Check sheet for the modelled part. Datum: model origin and axes. Units: mm. Face numbers are marked on the shaded views. A direction names the side the tool comes from. Round coordinates to 2 decimals unless told otherwise and drop trailing zeros. Write each loop counter-clockwise with the first axis right and the second up, starting at its lowest first coordinate (ties: lowest second). Pieces come first, ordered by that corner, then holes.
Item 1: Section check B-B, the plane z = -27. Record the cut outline in (x, y), plus the area to 3 significant figures.
Item 2: Section check C-C, the plane x = 15. Record the cut outline in (y, z).
Item 3: Depth check by flat-ended pin: pin 1 (1.2 mm diameter, centred on x = 7, y = 0.5, fed in from -Z); pin 2 (4 mm diameter, centred on x = -18, z = 5, fed in from +Y); pin 3 (1 mm diameter, centred on y = 9.5, z = -1.5, fed in from -X). Enter the tip coordinate at first touch or a pass-through.
Item 4: Material ranges on line 1 along Y through (x, z) = (0, 16); line 2 along Y through (x, z) = (-47, -10.5); line 3 along Z through (x, y) = (-6, 21.25), recorded low to high.
Item 5: Release check for a two-part mould opening along X. For the marked faces 3, 4, 5 and 6 record: pulls with the +X half, pulls with the -X half, needs draft (parallel to the pull), parting line crosses it, or undercut.
Item 6: Section check D-D, the plane y = 25.75. Record the cut outline in (x, z), plus the area to 3 significant figures.
Item 7: Section check A-A, the plane x = 0. Record the cut outline in (y, z).
Item 8: Set-up check for the marked faces 1 and 2: record each of +Z, -Z, +X, -X, +Y, -Y from which the full face is reachable in a straight line by a thin tool's end or side.
from build123d import *

# Parameters (mm, degrees)
SALIENTE_EXTRUIR1_DEPTH = 1.5
SALIENTE_EXTRUIR2_DEPTH = 30
CROQUIS3_R              = 8.9
CORTAR_EXTRUIR1_DEPTH   = 30
CROQUIS4_R              = 8.9
CORTAR_EXTRUIR2_DEPTH   = 30
CROQUIS5_R              = 8.9
CORTAR_EXTRUIR3_DEPTH   = 30


with BuildPart() as part:
    # Croquis1 → Saliente-Extruir1 (new body)
    with BuildSketch(Plane(origin=(0, 0, 0), x_dir=(1, 0, 0), z_dir=(0, 1, 0))):
        Polygon((-19, -15), (-51.571428571, 4.572992638), (-36.119065962, 30.287278353), (-19, 20), (-19, 15), (19, 15), (19, 20), (36.119065962, 30.287278353), (51.571428571, 4.572992638), (19, -15), align=None)
    extrude(amount=SALIENTE_EXTRUIR1_DEPTH)

    # Croquis2 → Saliente-Extruir2 (add)
    with BuildSketch(Plane(origin=(0, 0, 0), x_dir=(1, 0, 0), z_dir=(0, 1, 0))):
        Polygon((-51.571428571, 4.572992638), (-52.344046702, 3.287278353), (-19.416025147, -16.5), (19.416025147, -16.5), (52.344046702, 3.287278353), (51.571428571, 4.572992638), (19, -15), (-19, -15), align=None)
    extrude(amount=SALIENTE_EXTRUIR2_DEPTH)

    # Croquis3 → Cortar-Extruir1 (cut)
    with BuildSketch(Plane.XY.offset(16.5)):
        with Locations((0, 14.563888597)):
            Circle(CROQUIS3_R)
    extrude(amount=-CORTAR_EXTRUIR1_DEPTH, mode=Mode.SUBTRACT)

    # Croquis4 → Cortar-Extruir2 (cut)
    with BuildSketch(Plane(origin=(12.435875575, 0, 20.694547865), x_dir=(0.8571428571428564, 0, -0.5150787536377139), z_dir=(0.5150787536377139, 0, 0.8571428571428564))):
        with Locations((27.351520408, 15)):
            Circle(CROQUIS4_R)
    extrude(amount=-CORTAR_EXTRUIR2_DEPTH, mode=Mode.SUBTRACT)

    # Croquis5 → Cortar-Extruir3 (cut)
    with BuildSketch(Plane(origin=(-12.435875575, 0, 20.694547865), x_dir=(0.8571428571428567, 0, 0.5150787536377137), z_dir=(-0.5150787536377136, 0, 0.8571428571428565))):
        with Locations((-27.351520408, 15)):
            Circle(CROQUIS5_R)
    extrude(amount=-CORTAR_EXTRUIR3_DEPTH, mode=Mode.SUBTRACT)


solid = part.part
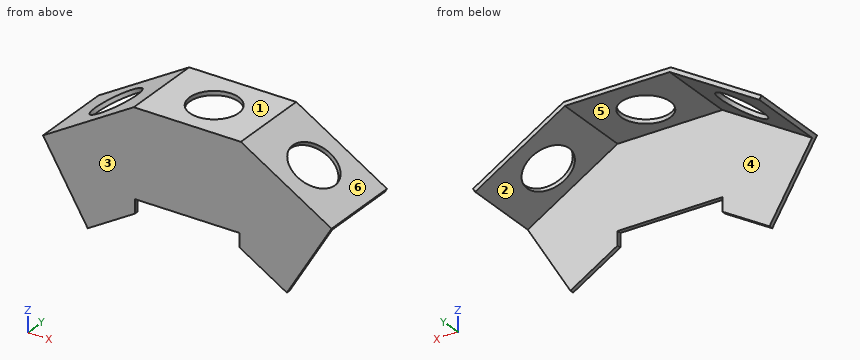
Values found:
1. outline: (-38.09, 0) - (-30.65, 0) - (-30.65, 1.5) - (-38.09, 1.5) - close; (30.65, 0) - (38.09, 0) - (38.09, 1.5) - (30.65, 1.5) - close
1. area: 22.3 mm2
2. outline: (0, -15) - (1.5, -15) - (1.5, 15) - (30, 15) - (30, 16.5) - (0, 16.5) - close
3. pin 1: stops at z = -15
3. pin 2: stops at y = 1.5
3. pin 3: stops at x = -50.2
4. line 1: y = 0 to 5.66, 23.46 to 30
4. line 2: y = 0 to 1.5
4. line 3: z = 15 to 16.5
5. face 3: needs draft
5. face 4: undercut
5. face 5: undercut
5. face 6: pulls with the +X half
6. outline: (-52.34, -3.29) - (-51.57, -4.57) - (-19, 15) - (19, 15) - (51.57, -4.57) - (52.34, -3.29) - (19.42, 16.5) - (-19.42, 16.5) - close
6. area: 172 mm2
7. outline: (0, -15) - (1.5, -15) - (1.5, 15) - (5.66, 15) - (5.66, 16.5) - (0, 16.5) - close; (23.46, 15) - (30, 15) - (30, 16.5) - (23.46, 16.5) - close
8. face 1: +Z, +X, -X, +Y, -Y
8. face 2: -Z, +Y
